from build123d import *

# Parameters (mm, degrees)
F0_W     = 0.2
F0_H     = 10
F0_W_2   = 2.9
F0_W_3   = 2.6
F0_W_4   = 2.3
F0_W_5   = 2
F0_W_6   = 1.7
F0_W_7   = 1.4
F0_W_8   = 0.8
F1_DEPTH = 5


with BuildPart() as f1:
    # F0 (on Top) → F1 (new body)
    with BuildSketch(Plane.XY):
        with Locations((-34.0027, -25)):
            Rectangle(F0_W, F0_H)
        Polygon((-33.9027, -30), (-34.1027, -30), (-34.1027, -32.4), (-0.786174, -32.4), (-0.786174, -30), (-3.686174, -30), (-5.454433, -30), (-8.054433, -30), (-11.126836, -30), (-13.426836, -30), (-16.084759, -30), (-18.084759, -30), (-20.736083, -30), (-22.436083, -30), (-25.499359, -30), (-26.899359, -30), (-30.313995, -30), (-31.113995, -30), align=None)
        Polygon((-34.2027, -20), (-34.1027, -20), (-33.9027, -20), (-33.8027, -20), (-33.8027, -10), (-34.2027, -10), align=None)
        Polygon((-34.3027, -10), (-34.2027, -10), (-33.8027, -10), (-33.7027, -10), (-33.7027, 0), (-34.3027, 0), align=None)
        with Locations((-2.236174, -25)):
            Rectangle(F0_W_2, F0_H)
        Polygon((-3.686174, -20), (-0.786174, -20), (-0.736174, -20), (-0.736174, -10), (-3.736174, -10), (-3.736174, -20), align=None)
        Polygon((-34.3027, 2.4), (-34.3027, 0), (-33.7027, 0), (-31.313995, 0), (-30.113995, 0), (-26.999359, 0), (-25.399359, 0), (-22.536083, 0), (-20.636083, 0), (-18.184759, 0), (-15.984759, 0), (-13.526836, 0), (-11.026836, 0), (-8.154433, 0), (-5.354433, 0), (-3.786174, 0), (-0.686174, 0), (-0.686174, 2.4), align=None)
        Polygon((-3.736174, -10), (-0.736174, -10), (-0.686174, -10), (-0.686174, 0), (-3.786174, 0), (-3.786174, -10), align=None)
        Polygon((-31.313995, -10), (-31.213995, -10), (-30.213995, -10), (-30.113995, -10), (-30.113995, 0), (-31.313995, 0), align=None)
        Polygon((-26.999359, -10), (-26.949359, -10), (-25.449359, -10), (-25.399359, -10), (-25.399359, 0), (-26.999359, 0), align=None)
        Polygon((-22.536083, -10), (-22.486083, -10), (-20.686083, -10), (-20.636083, -10), (-20.636083, 0), (-22.536083, 0), align=None)
        Polygon((-18.184759, -10), (-18.134759, -10), (-16.034759, -10), (-15.984759, -10), (-15.984759, 0), (-18.184759, 0), align=None)
        Polygon((-13.476836, -10), (-11.076836, -10), (-11.026836, -10), (-11.026836, 0), (-13.526836, 0), (-13.526836, -10), align=None)
        Polygon((-8.104433, -10), (-5.404433, -10), (-5.354433, -10), (-5.354433, 0), (-8.154433, 0), (-8.154433, -10), align=None)
        with Locations((-6.754433, -25)):
            Rectangle(F0_W_3, F0_H)
        with Locations((-12.276836, -25)):
            Rectangle(F0_W_4, F0_H)
        Polygon((-13.426836, -20), (-11.126836, -20), (-11.076836, -20), (-11.076836, -10), (-13.476836, -10), (-13.476836, -20), align=None)
        Polygon((-18.134759, -20), (-18.084759, -20), (-16.084759, -20), (-16.034759, -20), (-16.034759, -10), (-18.134759, -10), align=None)
        with Locations((-17.084759, -25)):
            Rectangle(F0_W_5, F0_H)
        with Locations((-21.586083, -25)):
            Rectangle(F0_W_6, F0_H)
        Polygon((-22.486083, -20), (-22.436083, -20), (-20.736083, -20), (-20.686083, -20), (-20.686083, -10), (-22.486083, -10), align=None)
        Polygon((-26.949359, -20), (-26.899359, -20), (-25.499359, -20), (-25.449359, -20), (-25.449359, -10), (-26.949359, -10), align=None)
        with Locations((-26.199359, -25)):
            Rectangle(F0_W_7, F0_H)
        Polygon((-31.213995, -20), (-31.113995, -20), (-30.313995, -20), (-30.213995, -20), (-30.213995, -10), (-31.213995, -10), align=None)
        with Locations((-30.713995, -25)):
            Rectangle(F0_W_8, F0_H)
        Polygon((-8.054433, -20), (-5.454433, -20), (-5.404433, -20), (-5.404433, -10), (-8.104433, -10), (-8.104433, -20), align=None)
    extrude(amount=F1_DEPTH)


solid = f1.part
Geometry: final body of the model. Coordinates: model frame, mm. Coordinates: 2 decimals unless noted, no trailing zeros. Write each loop counter-clockwise with the first axis right and the second up, starting at its lowest first coordinate (ties: lowest second). Pieces come first, ordered by that corner, then holes. Notation, with made-up numbers: (48, 52.25) - (100, 52.25) arc R26 cw to (100, 72.25) - close; hole circle Ø9 at (13, 70). An arc over 180 degrees is marked (long way). Return JSON: item names as keys, results as strings.
Item 1: Pin query (flat end, axial travel): pin 1 Ø2.5 at (y, z) = (-16.5, 2.5) entering from -X; pin 2 Ø1.5 at (y, z) = (-26.5, 2.5) entering from +X. Return the tip coordinate at first contact, or that it passes through.
Completed:
{"pin 1": "stops at x = -34.2", "pin 2": "stops at x = -0.79"}
Item 2: Line query: L1, parallel to Y at x = -32.5, z = 3.85. Output: solid intervals per line, ascending.
Completed:
{"L1": "y = -32.4 to -30, 0 to 2.4"}
Item 3: Section query A-A (x = -19). Output: boundary loops of the cut face in (y, z), and give its area (3 significant figures).
Completed:
{"outline": "(-32.4, 0) - (-30, 0) - (-30, 5) - (-32.4, 5) - close; (0, 0) - (2.4, 0) - (2.4, 5) - (0, 5) - close", "area": "24.0 mm2"}
Item 4: Section query B-B (y = -15). Count the separate pieces of the cut face and the enclosed holes in it, and give its area (3 significant figures).
Completed:
{"separate pieces": "8", "enclosed holes": "0", "area": "74.5 mm2"}
Item 5: Pull-direction query (X, two-part tool) for faces 1 (the face through (-5.354, -5, 2)), 2 (the face through (-34.103, -26, 2)), 3 (the face through (-16.035, -15, 2)), 4 (the face through (-0.786, -26, 2)); classes: +X half, -X half, draft (parallel to the pull), parting line (faces both ways), or undercut.
Completed:
{"face 1": "undercut", "face 2": "-X half", "face 3": "undercut", "face 4": "+X half"}
